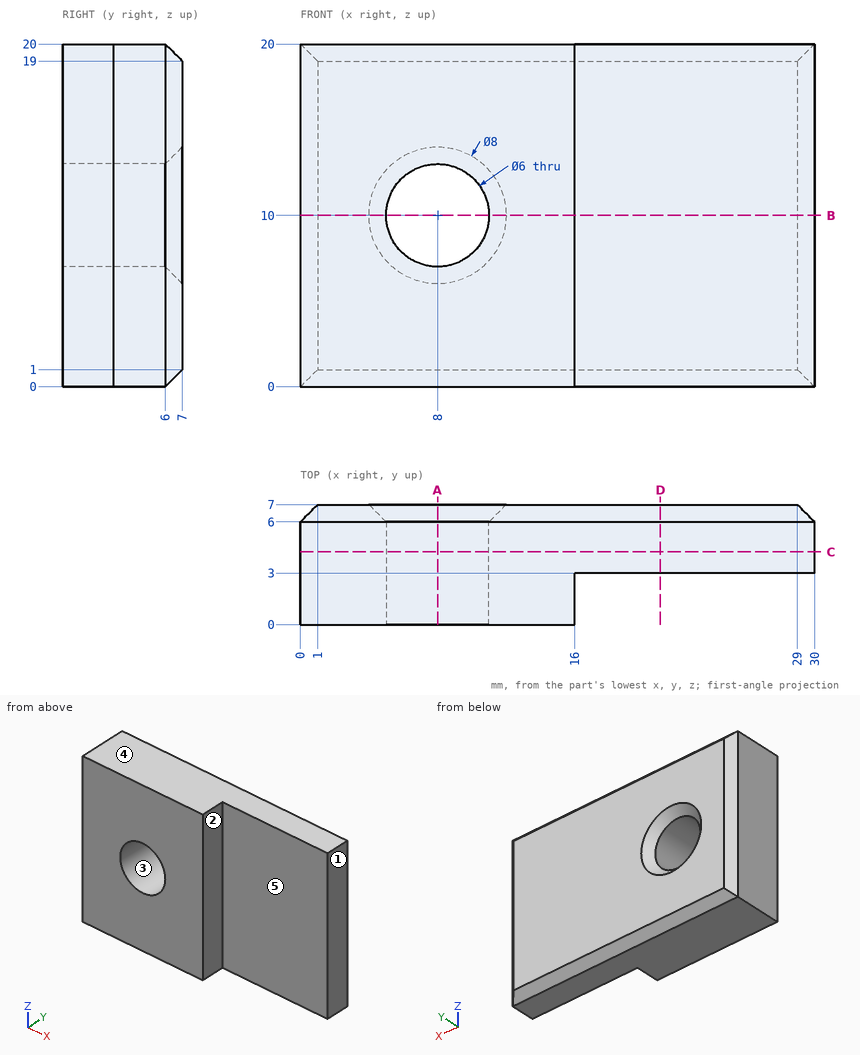
Can you work these out from the drawing? Everything is in mm from the part's minimum corner. A direction names the side the tool comes from. Give positions to 0.01 mm unless a question says otherwise; leave off trailing zeros. Order: outer loops, then holes, each group sorted by start corner. A loop starts at its lowest first (then second) coordinate and runs counter-clockwise, first axis right, second up.
Item 1: If we section it at C-C, the plane y = 4.25: Write out the boundary of the cut face in (x, z).
Item 2: If we section it at B-B, the plane z = 10: Write out the boundary of the cut face in (x, y), plus the area to 3 significant figures.
Item 3: If we mould it in two halves opening along Z, with no side actions, what happens to the marked faces 3, 4 and 5? For each: pulls with the +Z half, pulls with the -Z half, needs draft (parallel to the pull), parting line crosses it, or undercut.
Item 4: I need wall thicknesses on line 1 (X direction, y = 3.6, z = 10); line 2 (X direction, y = 2.8, z = 10); line 3 (Z direction, x = 8, y = 2.25). Which ranges of each line are inside material? Lowest first, please.
Item 5: For the marked faces 1 and 2, which set-ups out of +Z, -Z, +X, -X, +Y, -Y let a thin tool reach every point of the face, with its end or its side?
Item 6: I'm going to push flat-ended pins straight in: pin 1 (3.5 mm diameter, centred on y = 1, z = 12.5, fed in from +X); pin 2 (4 mm diameter, centred on x = 26.5, z = 12, fed in from -Y). Where does each tip first touch, or does it pass through?
Item 7: If we section it at A-A, the plane x = 8: Write out the boundary of the cut face in (y, z), plus the area to 3 significant figures.
Item 8: If we section it at D-D, the plane x = 21: Write out the boundary of the cut face in (y, z).
Values:
1. outline: (0, 0) - (30, 0) - (30, 20) - (0, 20) - close; hole circle Ø6 at (8, 10)
2. outline: (0, 0) - (5, 0) - (5, 6) - (4, 7) - (1, 7) - (0, 6) - close; (11, 0) - (16, 0) - (16, 3) - (30, 3) - (30, 6) - (29, 7) - (12, 7) - (11, 6) - close
2. area: 124 mm2
3. face 3: undercut
3. face 4: pulls with the +Z half
3. face 5: needs draft
4. line 1: x = 0 to 5, 11 to 30
4. line 2: x = 0 to 5, 11 to 16
4. line 3: z = 0 to 7, 13 to 20
5. face 1: +Z, -Z, +X, +Y, -Y
5. face 2: +Z, -Z, +X, -Y
6. pin 1: stops at x = 16
6. pin 2: stops at y = 3
7. outline: (0, 0) - (6, 0) - (7, 1) - (7, 6) - (6, 7) - (0, 7) - close; (0, 13) - (6, 13) - (7, 14) - (7, 19) - (6, 20) - (0, 20) - close
7. area: 96.0 mm2
8. outline: (3, 0) - (6, 0) - (7, 1) - (7, 19) - (6, 20) - (3, 20) - close
